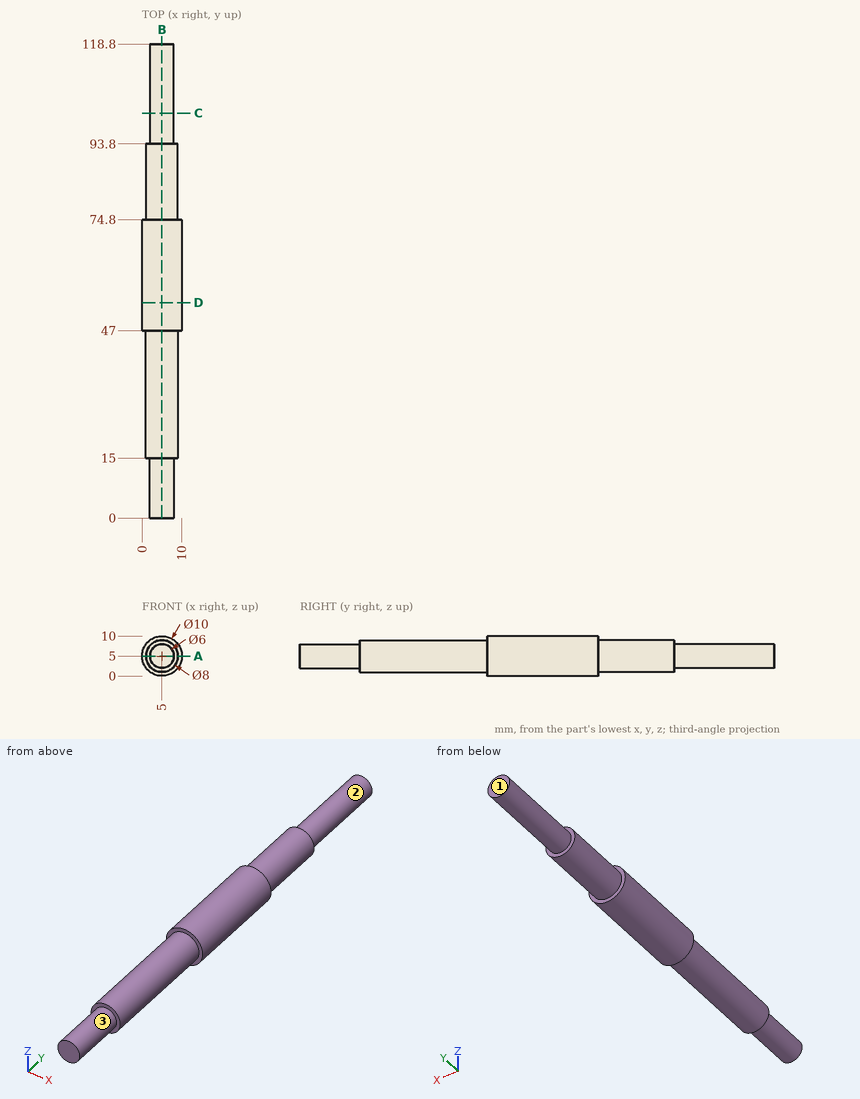
Print and shaded views of the part. All mm, measured from the part's lowest x, y and z. A direction names the side the tool comes from. Round coordinates to 2 decimals unless told otherwise and drop trailing zeros. Loops run counter-clockwise (first coordinate to the right, second up) from the corner with the lowest first, then second, coordinate; pieces in that order, holes last. Notation, with made-up numbers: M 5.25,80.5 L 13.25,80.5 A30 cw 13.25,118.5 Z; hole C 72,16 d7. An arc over 180 degrees is marked long. One line per question, with ' | ' between items.
1) Band-saw the part on B-B (x = 5). Give the cut face in (y, z).
Solved:
outline: M 0,2 L 15,2 L 15,1 L 47,1 L 47,0 L 74.8,0 L 74.8,1 L 93.8,1 L 93.8,2 L 118.8,2 L 118.8,8 L 93.8,8 L 93.8,9 L 74.8,9 L 74.8,10 L 47,10 L 47,9 L 15,9 L 15,8 L 0,8 Z
2) Flat gauge pins, fed straight in: pin 1 (3 mm diameter, centred on x = 1.5, z = 7, fed in from -Y); pin 2 (1 mm diameter, centred on y = 93, z = 5, fed in from +X). Where does each tip first touch, or does it go through?
Solved:
pin 1: stops at y = 0 | pin 2: stops at x = 9
3) Band-saw the part on A-A (z = 5). Give the cut face in (x, y).
Solved:
outline: M 0,47 L 1,47 L 1,15 L 2,15 L 2,0 L 8,0 L 8,15 L 9,15 L 9,47 L 10,47 L 10,74.8 L 9,74.8 L 9,93.8 L 8,93.8 L 8,118.8 L 2,118.8 L 2,93.8 L 1,93.8 L 1,74.8 L 0,74.8 Z
4) 3-axis set-ups, long thin cutter, end or side, ignore diameter. For the marked faces 1, 2 and 3: which of +Z, -Z, +X, -X, +Y, -Y reach the whole face in a straight line?
Solved:
face 1: +Z, -Z, +X, -X, +Y | face 2: +Y | face 3: -Y
5) Drill centre lines: line 1 along Z through (x, y) = (5, 102); line 2 along Y through (x, z) = (6.25, 8.5); line 3 along Z through (x, y) = (5, 22). Where is each one in solid material? Low to high.
Solved:
line 1: z = 2 to 8 | line 2: y = 15 to 93.8 | line 3: z = 1 to 9
6) Band-saw the part on C-C (y = 101.5). Give the cut face in (x, z).
Solved:
outline: C 5,5 d6
7) Band-saw the part on D-D (y = 54). Give the cut face in (x, z).
Solved:
outline: C 5,5 d10
